Part print with two shaded views. Sizes in mm from the minimum x, y, z corner. A direction names the side the tool comes from. Coordinates: 2 decimals unless noted, no trailing zeros. Write each loop counter-clockwise with the first axis right and the second up, starting at its lowest first coordinate (ties: lowest second). Pieces come first, ordered by that corner, then holes. Notation, with made-up numbers: (76.5, 40.25) -> (113.5, 40.25) arc R10 ccw to (113.5, 57.25) -> close; hole circle Ø2 at (84, -31). An arc over 180 degrees is marked (long way). Write item = value, one per line. Start each with the question number.
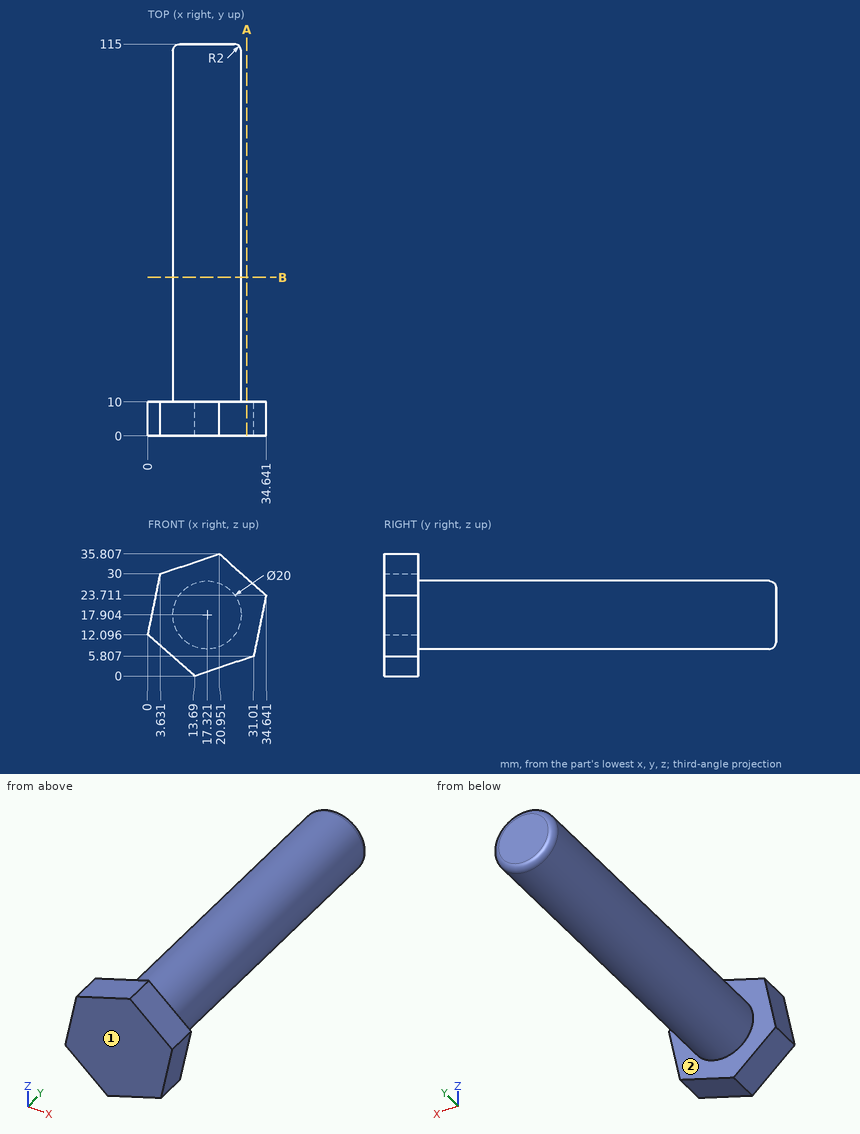
(1) Drill centre lines: line 1 along Y through (x, z) = (14.5, 31); line 2 along Z through (x, y) = (25, 108); line 3 along X through (y, z) = (31, 13) (1 decimal). Where is each one in solid material? Low to high.
(2) 3-axis set-ups, long thin cutter, end or side, ignore diameter. For the marked faces 1 and 2: which of +Z, -Z, +X, -X, +Y, -Y reach the whole face in a straight line?
(3) Saw through at B-B (y = 46.5). Give the cut face in (x, z).
(4) Drop flat-ended pins along their axis: pin 1 Ø4 at (x, y) = (28, 71.5) entering from -Z (1 decimal); pin 2 Ø5 at (x, y) = (18, 101.5) entering from +Z; pin 3 Ø1 at (y, z) = (75.5, 12) entering from +X (1 decimal). Give the stop position or say it passes through.
(5) Saw through at A-A (x = 29). Give the cut face in (y, z) (1 decimal), then the cut area to 3 significant figures.
Returned:
q1.line_1 = 0 to 10
q1.line_2 = 11.5 to 24.31
q1.line_3 = 8.6 to 26
q2.face_1 = +Z, -Z, +X, -X, -Y
q2.face_2 = +Y
q3.outline = circle Ø20 at (17.32, 17.9)
q4.pin_1 = 12.9
q4.pin_2 = 27.9
q4.pin_3 = 25.7
q5.outline = (0, 5.1) -> (10, 5.1) -> (10, 28.7) -> (0, 28.7) -> close
q5.area = 236 mm2
